Autodesk Inventor part; units mm, degrees
ref_plane "YZ Plane" through (0, 0, 0) normal (1, 0, 0) x (0, 1, 0)
ref_plane "XZ Plane" through (0, 0, 0) normal (0, 1, 0) x (-1, 0, 0)
ref_plane "XY Plane" through (0, 0, 0) normal (0, 0, 1) x (1, 0, 0)
sketch "Sketch1" plane through (0, 0, 0) normal (0, 0, 1) x (1, 0, 0)
  line L0 (0, 0) -> (201.5998, 0)
  line L1 (201.5998, 0) -> (201.5998, 63.754)
  line L2 (201.5998, 63.754) -> (0, 63.754)
  line L3 (0, 63.754) -> (0, 0)
  line L4 (0, 41.8592) -> (3.7465, 41.8592)
  line L5 (3.7465, 41.8592) -> (3.7465, 21.8948)
  line L6 (3.7465, 21.8948) -> (0, 21.8948)
  line L7 (0, 21.8948) -> (0, 41.8592)
  line L8 (201.5998, 41.8592) -> (197.8533, 41.8592)
  line L9 (197.8533, 41.8592) -> (197.8533, 21.8948)
  line L10 (197.8533, 21.8948) -> (201.5998, 21.8948)
  line L11 (201.5998, 21.8948) -> (201.5998, 41.8592)
  circle A0 centre (5.0546, 49.1744) radius 1.9558
  circle A1 centre (5.0546, 14.5796) radius 1.9558
  circle A2 centre (196.5452, 14.5796) radius 1.9558
  circle A3 centre (196.5452, 49.1744) radius 1.9558
  dimension "d0" = 201.5998
  dimension "d1" = 63.754
  dimension "d2" = 3.7465
  dimension "d3" = 19.9644
  dimension "d4" = 21.8948
  dimension "d5" = 3.7465
  dimension "d6" = 3.9116
  dimension "d7" = 12.6238
  dimension "d8" = 3.0988
  dimension "d9" = 3.9116
  dimension "d10" = 12.6238
  dimension "d11" = 3.0988
  dimension "d12" = 3.9116
  dimension "d13" = 3.0988
extrude "Extrusion1" add sketch "Sketch1" along normal blind 1.8796 contours L3 L6 L5 L4 L2 L1 L8 L9 L10 L0
fillet "Fillet1" radius 6.35 4 edges at (201.5998, 63.754, 0.9398) (201.5998, 0, 0.9398) (0, 63.754, 0.9398) (0, 0, 0.9398)
sketch "Sketch2" plane through (0, 0, 1.8796) normal (0, 0, 1) x (1, 0, 0)
  arc A0 (0, 6.35) -> (6.35, 0) centre (6.35, 6.35) ccw
  line L0 (6.35, 0) -> (195.2498, 0)
  arc A1 (195.2498, 0) -> (201.5998, 6.35) centre (195.2498, 6.35) ccw
  line L1 (201.5998, 6.35) -> (201.5998, 21.8948)
  line L2 (201.5998, 21.8948) -> (197.8533, 21.8948)
  line L3 (197.8533, 21.8948) -> (197.8533, 41.8592)
  line L4 (197.8533, 41.8592) -> (201.5998, 41.8592)
  line L5 (201.5998, 41.8592) -> (201.5998, 57.404)
  arc A2 (201.5998, 57.404) -> (195.2498, 63.754) centre (195.2498, 57.404) ccw
  line L6 (195.2498, 63.754) -> (6.35, 63.754)
  arc A3 (6.35, 63.754) -> (0, 57.404) centre (6.35, 57.404) ccw
  line L7 (0, 57.404) -> (0, 41.8592)
  line L8 (0, 41.8592) -> (3.7465, 41.8592)
  line L9 (3.7465, 41.8592) -> (3.7465, 21.8948)
  line L10 (3.7465, 21.8948) -> (0, 21.8948)
  line L11 (0, 21.8948) -> (0, 6.35)
  circle A4 centre (196.5452, 49.1744) radius 1.9558
  circle A5 centre (196.5452, 14.5796) radius 1.9558
  circle A6 centre (5.0546, 14.5796) radius 1.9558
  circle A7 centre (5.0546, 49.1744) radius 1.9558
  line L12 (15.0622, 60.5663) -> (170.4927, 60.5663)
  line L13 (170.4927, 60.5663) -> (170.4927, 9.7663)
  line L14 (15.0622, 9.7663) -> (15.0622, 60.5663)
  line L15 (170.4927, 9.7663) -> (170.4927, 6.5913)
  line L16 (26.4922, 6.5913) -> (26.4922, 9.7663)
  line L17 (159.5247, 6.5913) -> (159.5247, 3.4163)
  line L18 (159.5247, 3.4163) -> (42.0497, 3.4163)
  line L19 (42.0497, 3.4163) -> (42.0497, 6.5913)
  circle A8 centre (21.4122, 54.2163) radius 1.651
  circle A9 centre (21.4122, 16.129) radius 1.651
  circle A10 centre (165.0087, 16.129) radius 1.651
  circle A11 centre (165.0087, 54.2163) radius 1.651
  line L20 (33.3756, 50.5714) -> (117.4496, 50.5714)
  line L21 (117.4496, 50.5714) -> (117.4496, 28.8544)
  line L22 (117.4496, 28.8544) -> (33.3756, 28.8544)
  line L23 (33.3756, 28.8544) -> (33.3756, 50.5714)
  line L24 (39.2811, 23.114) -> (50.0761, 23.114)
  line L25 (50.0761, 23.114) -> (50.0761, 12.319)
  line L26 (50.0761, 12.319) -> (39.2811, 12.319)
  line L27 (39.2811, 12.319) -> (39.2811, 23.114)
  line L28 (54.6481, 23.114) -> (65.4431, 23.114)
  line L29 (65.4431, 23.114) -> (65.4431, 12.319)
  line L30 (65.4431, 12.319) -> (54.6481, 12.319)
  line L31 (54.6481, 12.319) -> (54.6481, 23.114)
  line L32 (70.0151, 23.114) -> (80.8101, 23.114)
  line L33 (80.8101, 23.114) -> (80.8101, 12.319)
  line L34 (80.8101, 12.319) -> (70.0151, 12.319)
  line L35 (70.0151, 12.319) -> (70.0151, 23.114)
  line L36 (85.3821, 23.114) -> (96.1771, 23.114)
  line L37 (96.1771, 23.114) -> (96.1771, 12.319)
  line L38 (96.1771, 12.319) -> (85.3821, 12.319)
  line L39 (85.3821, 12.319) -> (85.3821, 23.114)
  line L40 (100.7491, 23.114) -> (111.5441, 23.114)
  line L41 (111.5441, 23.114) -> (111.5441, 12.319)
  line L42 (111.5441, 12.319) -> (100.7491, 12.319)
  line L43 (100.7491, 12.319) -> (100.7491, 23.114)
  line L44 (138.7221, 23.114) -> (149.5171, 23.114)
  line L45 (149.5171, 23.114) -> (149.5171, 12.319)
  line L46 (149.5171, 12.319) -> (138.7221, 12.319)
  line L47 (138.7221, 12.319) -> (138.7221, 23.114)
  line L48 (170.4927, 9.7663) -> (170.4927, 9.7663)
  line L49 (26.4922, 9.7663) -> (15.0622, 9.7663)
  line L50 (26.4922, 6.5913) -> (42.0497, 6.5913)
  line L51 (159.5247, 6.5913) -> (170.4927, 6.5913)
  circle A12 centre (176.1998, 40.132) radius 4.2799
  circle A13 centre (176.1998, 23.622) radius 4.2799
  circle A14 centre (144.1196, 41.5163) radius 3.4925
  line L52 (144.1196, 23.114) -> (144.1196, 12.319)
  point P0 (0, 0)
  dimension "d30" = 3.302
  dimension "d31" = 6.35
  dimension "d32" = 6.35
  dimension "d42" = 84.074
  dimension "d43" = 21.717
  dimension "d72" = 10.795
  dimension "d73" = 10.795
  dimension "d74" = 10.795
  dimension "d75" = 10.795
  dimension "d76" = 10.795
  dimension "d77" = 10.795
  dimension "d78" = 10.795
  dimension "d79" = 4.572
  dimension "d80" = 4.572
  dimension "d81" = 4.572
  dimension "d82" = 4.572
  dimension "d83" = 5.9055
  dimension "d84" = 5.9055
  dimension "d85" = 12.319
  dimension "d86" = 8.5598
  dimension "d87" = 8.5598
  dimension "d90" = 6.985
  dimension "d91" = 26.67
  dimension "d99" = 25.4
  dimension "d100" = 25.4
  dimension "d101" = 0
  dimension "d102" = 3.302
  dimension "d103" = 3.302
  dimension "d104" = 3.302
  dimension "d106" = 16.51
  dimension "d108" = 23.622
  dimension "d109" = 23.622
  dimension "d112" = 50.8
  dimension "d113" = 155.4305
  dimension "d114" = 6.35
extrude "Extrusion2" cut sketch "Sketch2" against normal blind 1.8796 contours A8 | A9 | A10 | A11 | L20 L21 L22 L23 | L24 L25 L26 L27 | L28 L29 L30 L31 | L32 L33 L34 L35 | L36 L37 L38 L39 | L40 L41 L42 L43 | L44 L52 L46 L47 | L44 L45 L46 L52 | A12 | A13 | A14
extrude "Extrusion3" add sketch "Sketch2" against normal blind 3.7592 contours L12 L13 L15 L51 L17 L18 L19 L50 L16 L49 L14
sketch "Sketch3" plane through (0, 0, 1.8796) normal (0, 0, 1) x (1, 0, 0)
  line L0 (138.7221, 12.319) -> (138.7221, 23.114)
  line L1 (138.7221, 23.114) -> (149.5171, 23.114)
  line L2 (149.5171, 23.114) -> (149.5171, 12.319)
  line L3 (149.5171, 12.319) -> (138.7221, 12.319)
  line L4 (85.3821, 12.319) -> (85.3821, 23.114)
  line L5 (85.3821, 23.114) -> (96.1771, 23.114)
  line L6 (96.1771, 23.114) -> (96.1771, 12.319)
  line L7 (96.1771, 12.319) -> (85.3821, 12.319)
  line L8 (54.6481, 12.319) -> (54.6481, 23.114)
  line L9 (54.6481, 23.114) -> (65.4431, 23.114)
  line L10 (65.4431, 23.114) -> (65.4431, 12.319)
  line L11 (65.4431, 12.319) -> (54.6481, 12.319)
  circle A0 centre (144.1196, 41.5163) radius 3.4925
  circle A1 centre (165.0087, 16.129) radius 1.651
  circle A2 centre (21.4122, 54.2163) radius 1.651
  circle A3 centre (21.4122, 16.129) radius 1.651
  circle A4 centre (165.0087, 54.2163) radius 1.651
  line L12 (39.2811, 12.319) -> (39.2811, 23.114)
  line L13 (39.2811, 23.114) -> (50.0761, 23.114)
  line L14 (50.0761, 23.114) -> (50.0761, 12.319)
  line L15 (50.0761, 12.319) -> (39.2811, 12.319)
  line L16 (70.0151, 12.319) -> (70.0151, 23.114)
  line L17 (70.0151, 23.114) -> (80.8101, 23.114)
  line L18 (80.8101, 23.114) -> (80.8101, 12.319)
  line L19 (80.8101, 12.319) -> (70.0151, 12.319)
  line L20 (100.7491, 12.319) -> (100.7491, 23.114)
  line L21 (100.7491, 23.114) -> (111.5441, 23.114)
  line L22 (111.5441, 23.114) -> (111.5441, 12.319)
  line L23 (111.5441, 12.319) -> (100.7491, 12.319)
  line L24 (33.3756, 28.8544) -> (33.3756, 50.5714)
  line L25 (33.3756, 50.5714) -> (117.4496, 50.5714)
  line L26 (117.4496, 50.5714) -> (117.4496, 28.8544)
  line L27 (117.4496, 28.8544) -> (33.3756, 28.8544)
  circle A5 centre (176.1998, 23.622) radius 4.2799
  circle A6 centre (176.1998, 40.132) radius 4.2799
  arc A7 (0, 6.35) -> (6.35, 0) centre (6.35, 6.35) ccw
  line L28 (6.35, 0) -> (195.2498, 0)
  arc A8 (195.2498, 0) -> (201.5998, 6.35) centre (195.2498, 6.35) ccw
  line L29 (201.5998, 6.35) -> (201.5998, 21.8948)
  line L30 (201.5998, 21.8948) -> (197.8533, 21.8948)
  line L31 (197.8533, 21.8948) -> (197.8533, 41.8592)
  line L32 (197.8533, 41.8592) -> (201.5998, 41.8592)
  line L33 (201.5998, 41.8592) -> (201.5998, 57.404)
  arc A9 (201.5998, 57.404) -> (195.2498, 63.754) centre (195.2498, 57.404) ccw
  line L34 (195.2498, 63.754) -> (6.35, 63.754)
  arc A10 (6.35, 63.754) -> (0, 57.404) centre (6.35, 57.404) ccw
  line L35 (0, 57.404) -> (0, 41.8592)
  line L36 (0, 41.8592) -> (3.7465, 41.8592)
  line L37 (3.7465, 41.8592) -> (3.7465, 21.8948)
  line L38 (3.7465, 21.8948) -> (0, 21.8948)
  line L39 (0, 21.8948) -> (0, 6.35)
  circle A11 centre (196.5452, 49.1744) radius 1.9558
  circle A12 centre (196.5452, 14.5796) radius 1.9558
  circle A13 centre (5.0546, 14.5796) radius 1.9558
  circle A14 centre (5.0546, 49.1744) radius 1.9558
  circle A15 centre (21.4122, 54.2163) radius 1.651
  line L40 (15.0622, 60.5663) -> (170.4927, 60.5663)
  line L41 (138.7221, 12.319) -> (138.7221, 23.114)
  line L42 (138.7221, 23.114) -> (149.5171, 23.114)
  line L43 (149.5171, 23.114) -> (149.5171, 12.319)
  line L44 (149.5171, 12.319) -> (138.7221, 12.319)
  line L45 (85.3821, 12.319) -> (85.3821, 23.114)
  line L46 (85.3821, 23.114) -> (96.1771, 23.114)
  line L47 (96.1771, 23.114) -> (96.1771, 12.319)
  line L48 (96.1771, 12.319) -> (85.3821, 12.319)
  line L49 (54.6481, 12.319) -> (54.6481, 23.114)
  line L50 (54.6481, 23.114) -> (65.4431, 23.114)
  line L51 (65.4431, 23.114) -> (65.4431, 12.319)
  line L52 (65.4431, 12.319) -> (54.6481, 12.319)
  circle A16 centre (144.1196, 41.5163) radius 3.4925
  circle A17 centre (165.0087, 16.129) radius 1.651
  circle A18 centre (21.4122, 54.2163) radius 1.651
  circle A19 centre (21.4122, 16.129) radius 1.651
  circle A20 centre (165.0087, 54.2163) radius 1.651
  line L53 (39.2811, 12.319) -> (39.2811, 23.114)
  line L54 (39.2811, 23.114) -> (50.0761, 23.114)
  line L55 (50.0761, 23.114) -> (50.0761, 12.319)
  line L56 (50.0761, 12.319) -> (39.2811, 12.319)
  line L57 (70.0151, 12.319) -> (70.0151, 23.114)
  line L58 (70.0151, 23.114) -> (80.8101, 23.114)
  line L59 (80.8101, 23.114) -> (80.8101, 12.319)
  line L60 (80.8101, 12.319) -> (70.0151, 12.319)
  line L61 (100.7491, 12.319) -> (100.7491, 23.114)
  line L62 (100.7491, 23.114) -> (111.5441, 23.114)
  line L63 (111.5441, 23.114) -> (111.5441, 12.319)
  line L64 (111.5441, 12.319) -> (100.7491, 12.319)
  line L65 (33.3756, 28.8544) -> (33.3756, 50.5714)
  line L66 (33.3756, 50.5714) -> (117.4496, 50.5714)
  line L67 (117.4496, 50.5714) -> (117.4496, 28.8544)
  line L68 (117.4496, 28.8544) -> (33.3756, 28.8544)
  circle A21 centre (176.1998, 23.622) radius 4.2799
  circle A22 centre (176.1998, 40.132) radius 4.2799
  arc A23 (0, 6.35) -> (6.35, 0) centre (6.35, 6.35) ccw
  line L69 (6.35, 0) -> (195.2498, 0)
  arc A24 (195.2498, 0) -> (201.5998, 6.35) centre (195.2498, 6.35) ccw
  line L70 (201.5998, 6.35) -> (201.5998, 21.8948)
  line L71 (201.5998, 21.8948) -> (197.8533, 21.8948)
  line L72 (197.8533, 21.8948) -> (197.8533, 41.8592)
  line L73 (197.8533, 41.8592) -> (201.5998, 41.8592)
  line L74 (201.5998, 41.8592) -> (201.5998, 57.404)
  arc A25 (201.5998, 57.404) -> (195.2498, 63.754) centre (195.2498, 57.404) ccw
  line L75 (195.2498, 63.754) -> (6.35, 63.754)
  arc A26 (6.35, 63.754) -> (0, 57.404) centre (6.35, 57.404) ccw
  line L76 (0, 57.404) -> (0, 41.8592)
  line L77 (0, 41.8592) -> (3.7465, 41.8592)
  line L78 (3.7465, 41.8592) -> (3.7465, 21.8948)
  line L79 (3.7465, 21.8948) -> (0, 21.8948)
  line L80 (0, 21.8948) -> (0, 6.35)
  circle A27 centre (196.5452, 49.1744) radius 1.9558
  circle A28 centre (196.5452, 14.5796) radius 1.9558
  circle A29 centre (5.0546, 14.5796) radius 1.9558
  circle A30 centre (5.0546, 49.1744) radius 1.9558
  circle A31 centre (21.4122, 54.2163) radius 1.651
  circle A32 centre (21.4122, 16.129) radius 1.651
  circle A33 centre (165.0087, 16.129) radius 1.651
  circle A34 centre (165.0087, 54.2163) radius 1.651
  point P0 (0, 0)
extrude "Extrusion4" add sketch "Sketch3" against normal blind 12.7 contours A1 | A2 | A3 | A4
properties part number "Front Pannel"
Work out the finished part from the listing and answer in its coordinate system (mm). A direction names the side the tool comes from. Round coordinates to 2 decimals unless told otherwise and drop trailing zeros. Write each loop counter-clockwise with the first axis right and the second up, starting at its lowest first coordinate (ties: lowest second). Pieces come first, ordered by that corner, then holes. Notation, with made-up numbers: M 71.25,40.25 L 86.25,40.25 A5 ccw 86.25,45.25 Z; hole C 72,-31.75 d3. An arc over 180 degrees is marked long. Use a Markdown table: item, result.
1) The part is cut by section A-A on x = 114. Give the vertices of the cut face in (y, z), plus the area to 3 significant figures.
Taken from the geometry:
| item | result |
|---|---|
| outline | M 0,0 L 3.42,0 L 3.42,-1.88 L 28.85,-1.88 L 28.85,1.88 L 0,1.88 Z; M 50.57,-1.88 L 60.57,-1.88 L 60.57,0 L 63.75,0 L 63.75,1.88 L 50.57,1.88 Z |
| area | 146 mm2 |
2) The part is cut by section D-D on x = 183. Give the vertices of the cut face in (y, z), plus the area to 3 significant figures.
Taken from the geometry:
| item | result |
|---|---|
| outline | M 0,0 L 63.75,0 L 63.75,1.88 L 0,1.88 Z |
| area | 120 mm2 |
3) Which of the six approach directions +Z, -Z, +X, -X, +Y, -Y give full straight-line access (tool end or side, diameter ignored) to faces 1 (the face through (21.197, 55.853, -6.287)), 2 (the face through (21, 16, -10.82)), 3 (the face through (85.382, 18, 0))?
Taken from the geometry:
| item | result |
|---|---|
| face 1 | -Z |
| face 2 | -Z, +X, -X, +Y, -Y |
| face 3 | +Z, -Z |
4) Determine the mould class of faces 4 (the face through (199.69, 1.81, 0.95)), 5 (the face through (21, 54, -10.82)), 6 (the face through (6.106, 12.93, 0.927)) for opening direction Y: pulls with the +Y half, pulls with the -Y half, needs draft (parallel to the pull), parting line crosses it, or undercut.
Taken from the geometry:
| item | result |
|---|---|
| face 4 | pulls with the -Y half |
| face 5 | needs draft |
| face 6 | undercut |
5) Flat-ended cylindrical pins translate along their axes: pin 1 (1.5 mm diameter, centred on x = 86, y = 29, fed in from -Z); pin 2 (1.5 mm diameter, centred on x = 32.5, z = -1, fed in from -Y); pin 3 (0.9 mm diameter, centred on y = 33.5, z = 0.5, fed in from -X). Find the tip coordinate at first contact, or state that the pin passes through.
Taken from the geometry:
| item | result |
|---|---|
| pin 1 | stops at z = -1.88 |
| pin 2 | stops at y = 6.59 |
| pin 3 | stops at x = 3.75 |
6) The part is cut by section B-B on x = 45. Give the vertices of the cut face in (y, z).
Taken from the geometry:
| item | result |
|---|---|
| outline | M 0,0 L 3.42,0 L 3.42,-1.88 L 12.32,-1.88 L 12.32,1.88 L 0,1.88 Z; M 23.11,-1.88 L 28.85,-1.88 L 28.85,1.88 L 23.11,1.88 Z; M 50.57,-1.88 L 60.57,-1.88 L 60.57,0 L 63.75,0 L 63.75,1.88 L 50.57,1.88 Z |
7) The part is cut by section C-C on z = -8. Give the vertices of the cut face in (x, y), plus the area to 3 significant figures.
Taken from the geometry:
| item | result |
|---|---|
| outline | C 21.41,16.13 d3.3; C 21.41,54.22 d3.3; C 165.01,16.13 d3.3; C 165.01,54.22 d3.3 |
| area | 34.3 mm2 |
8) Consider line 1 (Y direction, x = 88, z = -1.75); line 2 (Y direction, x = 61.5, z = 0.5); line 3 (X direction, y = 35.5, z = -1.75). Determine where each line is inside the solid, lowest interval first. Write a range as [from, to].
Taken from the geometry:
| item | result |
|---|---|
| line 1 | y = [3.42, 12.32], [23.11, 28.85], [50.57, 60.57] |
| line 2 | y = [0, 12.32], [23.11, 28.85], [50.57, 63.75] |
| line 3 | x = [15.06, 33.38], [117.45, 170.49] |
